```python
from build123d import *


with BuildPart() as part:
    # Sketch1 → Revolve1 (revolve)
    with BuildSketch(Plane.XY):
        with BuildLine():
            Line((-0.639512806, 9.167562806), (-0.381, 8.90905))
            Line((-0.381, 8.90905), (0, 8.90905))
            Line((0, 8.90905), (0.762, 9.67105))
            Line((0.762, 9.67105), (81.9277, 9.67105))
            Line((81.9277, 9.67105), (82.6897, 8.90905))
            Line((82.6897, 8.90905), (83.0707, 8.90905))
            Line((83.0707, 8.90905), (83.329212806, 9.167562806))
            ThreePointArc((83.329212806, 9.167562806), (83.366410245, 9.257365367), (83.329212806, 9.347167928))
            Line((83.329212806, 9.347167928), (82.644315367, 10.032065367))
            ThreePointArc((82.644315367, 10.032065367), (82.397104775, 10.197246204), (82.1055, 10.25525))
            Line((82.1055, 10.25525), (0.5842, 10.25525))
            ThreePointArc((0.5842, 10.25525), (0.292595225, 10.197246204), (0.045384633, 10.032065367))
            Line((0.045384633, 10.032065367), (-0.639512806, 9.347167928))
            ThreePointArc((-0.639512806, 9.347167928), (-0.676710245, 9.257365367), (-0.639512806, 9.167562806))
        make_face()
    revolve(axis=Axis((82.6897, 0, 0), (-1, 0, 0)))


solid = part.part
```
Geometry check sheet. Reference: the model listing, model coordinates, mm. A direction names the side the tool comes from. Coordinates: 2 decimals unless noted, no trailing zeros. Loops run counter-clockwise (first coordinate to the right, second up) from the corner with the lowest first, then second, coordinate; pieces in that order, holes last. Notation, with made-up numbers: (26.5, -28) -> (80.5, -28) arc R18 ccw to (80.5, -3) -> close; hole circle Ø1 at (58.5, -1.5). An arc over 180 degrees is marked (long way). Put each result on its own line as item: value.
1) Cross-section at A-A on y = 0. Record the boundary of the cut face in (x, z), plus the area to 3 significant figures.
Result set:
outline: (-0.64, -9.35) -> (0.05, -10.03) arc R0.76 ccw to (0.58, -10.26) -> (82.11, -10.26) arc R0.76 ccw to (82.64, -10.03) -> (83.33, -9.35) arc R0.13 ccw to (83.33, -9.17) -> (83.07, -8.91) -> (82.69, -8.91) -> (81.93, -9.67) -> (0.76, -9.67) -> (0, -8.91) -> (-0.38, -8.91) -> (-0.64, -9.17) arc R0.13 ccw to start; (-0.64, 9.17) -> (-0.38, 8.91) -> (0, 8.91) -> (0.76, 9.67) -> (81.93, 9.67) -> (82.69, 8.91) -> (83.07, 8.91) -> (83.33, 9.17) arc R0.13 ccw to (83.33, 9.35) -> (82.64, 10.03) arc R0.76 ccw to (82.11, 10.26) -> (0.58, 10.26) arc R0.76 ccw to (0.05, 10.03) -> (-0.64, 9.35) arc R0.13 ccw to start
area: 99.4 mm^2
2) Gauge pin test, flat ends, axial feed: pin 1 Ø5 at (x, y) = (11.5, 5.5) entering from -Z; pin 2 Ø12 at (x, y) = (39.5, 7.5) entering from +Z; pin 3 Ø4 at (x, y) = (22, -7.5) entering from -Z; pin 4 Ø1.5 at (y, z) = (-6.5, -3) entering from -X. Record the tip position at first contact, or that the pin passes through.
Result set:
pin 1: stops at z = -9.81
pin 2: stops at z = 10.14
pin 3: stops at z = -8.66
pin 4: passes through
3) Tool access check on faces 3 (the cylindrical face through (82.883, 8.498, -2.676)), 4 (the cylindrical face through (41.913, 9.224, -2.905)). Record the directions out of +Z, -Z, +X, -X, +Y, -Y that give a thin tool (end or side, any length) a straight path to the whole face; none if there is none.
Result set:
face 3: +X, -X
face 4: none
4) Release check for a two-part mould opening along Z. For faces 1 (the cylindrical face through (40.774, -2.223, 10.011)), 2 (the cylindrical face through (-0.188, 8.498, -2.676)) record: released by +Z, released by -Z, zero draft, split by the parting line, or undercut.
Result set:
face 1: split by the parting line
face 2: undercut
5) Cross-section at C-C on x = 30. Record the boundary of the cut face in (y, z).
Result set:
outline: circle Ø20.51 at (0, 0); hole circle Ø19.34 at (0, 0)
6) Thickness scan on line 1 (Y direction, x = 57, z = 0); line 2 (Z direction, x = 62.5, y = -0.5); line 3 (Z direction, x = 16, y = -5). Record the ranges inside material, lowest first.
Result set:
line 1: y = -10.26 to -9.67, 9.67 to 10.26
line 2: z = -10.24 to -9.66, 9.66 to 10.24
line 3: z = -8.95 to -8.28, 8.28 to 8.95
